For this review, take the finished solid that the model builds, in its own axes (mm). Face numbers are marked on the shaded views. A direction names the side the tool comes from. Round coordinates to 2 decimals unless told otherwise and drop trailing zeros. Order: outer loops, then holes, each group sorted by start corner. A loop starts at its lowest first (then second) coordinate and runs counter-clockwise, first axis right, second up. Notation, with made-up numbers: M 82,2.5 L 108,2.5 A16 cw 108,24.5 Z; hole C -23,79.25 d2. An arc over 180 degrees is marked long. Answer as a JSON object with one key per item and string values.
from build123d import *

# Parameters (mm, degrees)
BOSS_EXTRUDE3_DEPTH    = 370
SKETCH3_W              = 619.706220458
SKETCH3_H              = 524.5
BOSS_EXTRUDE4_DEPTH    = 50
BOSS_EXTRUDE6_DEPTH    = 420
CHAMFER1_SIZE          = 30
SHELL1_T               = -3.18
CUT_EXTRUDE1_DEPTH     = 10
BOSS_EXTRUDE7_REACH    = 652.082
SKETCH13_W             = 122.046220458
SKETCH13_H             = 233.985108613
CUT_EXTRUDE3_DEPTH     = 651.08233795
SPLIT2_SURFACE_1_BACK  = 938.174
SPLIT2_SURFACE_1_DEPTH = 1876.348
BOSS_EXTRUDE8_DEPTH    = 3.18


with BuildPart() as part:
    # Sketch1 → Boss-Extrude3 (new body)
    with BuildSketch(Plane(origin=(0, 0, 0), x_dir=(1, 0, 0), z_dir=(0, 1, 0))):
        Polygon((225.65, -262.25), (394.056220458, -262.25), (394.056220458, 262.25), (225.65, 262.25), (-225.65, 262.25), (-225.65, -262.25), align=None)
    extrude(amount=BOSS_EXTRUDE3_DEPTH)

    # Sketch3 → Boss-Extrude4 (add)
    with BuildSketch(Plane(origin=(0, 370, 0), x_dir=(1, 0, 0), z_dir=(0, 1, 0))):
        with Locations((84.203110229, 0)):
            Rectangle(SKETCH3_W, SKETCH3_H)
    extrude(amount=BOSS_EXTRUDE4_DEPTH)

    # Sketch9 → Boss-Extrude6 (add)
    with BuildSketch(Plane(origin=(0, 0, 0), x_dir=(1, 0, 0), z_dir=(0, 1, 0))):
        Polygon((-225.65, -262.25), (-152.747945688, -301.540612909), (321.154166146, -301.540612909), (394.056220458, -262.25), align=None)
    extrude(amount=BOSS_EXTRUDE6_DEPTH)

    # Chamfer1
    chamfer1_edges = [part.edges().sort_by_distance(p)[0] for p in [
        (-189.198972844, 420, 281.895306454),
        (84.203110229, 420, 301.540612909),
        (357.605193302, 420, 281.895306454),
    ]]
    chamfer(chamfer1_edges, length=CHAMFER1_SIZE)

    # Shell1
    shell1_openings = [part.faces().sort_by_distance(p)[0] for p in [
        (84.203110229, 0, 17.423394881),
    ]]
    offset(amount=SHELL1_T, openings=shell1_openings, kind=Kind.INTERSECTION)

    # Sketch7 → Cut-Extrude1 (cut)
    with BuildSketch(Plane.ZY.offset(225.65)):
        Polygon((-19.07, 315), (-19.07, 230), (20.93, 190), (80.93, 190), (120.93, 230), (120.93, 315), align=None)
    extrude(amount=-CUT_EXTRUDE1_DEPTH, mode=Mode.SUBTRACT)


with BuildPart() as body_2:

    # Sketch12 → Boss-Extrude7 (new, up to next)
    with BuildSketch(Plane(origin=(0, 0, 0), x_dir=(1, 0, 0), z_dir=(0, 1, 0)), mode=Mode.PRIVATE) as boss_extrude7_sk1:
        Polygon((225.65, -262.25), (225.65, -298.360612909), (320.351791074, -298.360612909), (390.876220458, -260.35142261), (390.876220458, 259.07), (225.65, 259.07), align=None)
    boss_extrude7_tool1 = extrude(boss_extrude7_sk1.sketch, amount=BOSS_EXTRUDE7_REACH, mode=Mode.PRIVATE) - part.part
    add(boss_extrude7_tool1.solids().sort_by_distance((307.390302, 0, 15.716589))[0])

    # Sketch13 → Cut-Extrude3 (cut, through all)
    with BuildSketch(Plane.XZ):
        with Locations((289.853110229, 233.456942929)):
            Rectangle(SKETCH13_W, SKETCH13_H)
    extrude(amount=-CUT_EXTRUDE3_DEPTH, mode=Mode.SUBTRACT)


with BuildPart() as part_1:
    add(part.part)

    # Split2: cut with a surface, the side it looks to stays
    # Split2 surface: a surface, the sketch's curves swept straight by 1876.348 mm
    with BuildLine(Plane.ZY.offset(225.65).offset(-SPLIT2_SURFACE_1_BACK), mode=Mode.PRIVATE) as split2_surface_1_path:
        Line((377.982656301, 50), (20.93, 50))
        Line((20.93, 50), (-30.817816509, 101.747816509))
        Line((-30.817816509, 101.747816509), (-303.707153017, 101.747816509))
    split2_surface_1 = Shell.extrude(split2_surface_1_path.wire(), (-1 * SPLIT2_SURFACE_1_DEPTH, 0 * SPLIT2_SURFACE_1_DEPTH, 0 * SPLIT2_SURFACE_1_DEPTH))
    split(bisect_by=split2_surface_1, keep=Keep.TOP)

    add(body_2.part)  # Boss-Extrude8 merges body 2
    # Sketch14 → Boss-Extrude8 (add)
    with BuildSketch(Plane.XZ):
        Polygon((394.056220458, 262.25), (394.056220458, -262.25), (-225.65, -262.25), (-225.65, 262.25), (-152.747945688, 301.540612909), (321.154166146, 301.540612909), align=None)
    extrude(amount=BOSS_EXTRUDE8_DEPTH)


solid = part_1.part
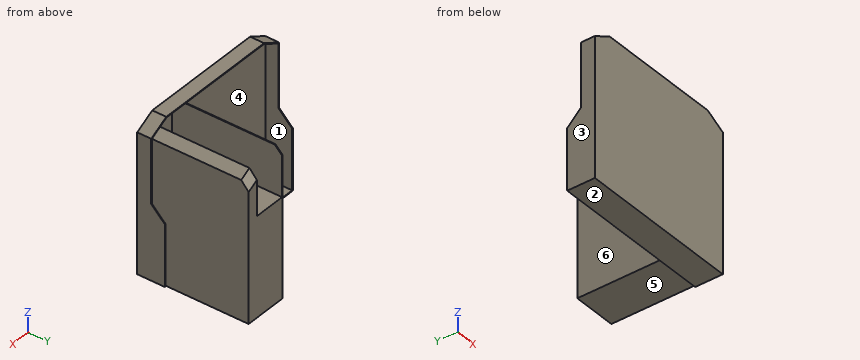
1) Add section B-B on z = 64. State the section outline as (x, y) points.
Geometry check:
{"outline": "M -225.65,-3.18 L 394.06,-3.18 L 394.06,50 L 390.88,50 L 390.88,416.82 L 225.65,416.82 L 225.65,0 L -222.47,0 L -222.47,50 L -225.65,50 Z"}
2) Machinability: for the marked faces 1 and 2, which of the approach directions +Z, -Z, +X, -X, +Y, -Y give a long, thin tool a straight path to every point of the face, cutting with its end or side? Answer none if there is none.
Geometry check:
{"face 1": "+Y", "face 2": "-Z, +X, -X, +Y, -Y"}
3) For L1, parallel to Z at x = 65, y = 19.5; L2, parallel to X at y = 36, z = -109.5; L3, parallel to Z at x = -33, y = 71, list the stretches that pass through material, from the lowest coordinate up.
Geometry check:
{"L1": "z = -262.25 to -259.07, 298.36 to 301.54", "L2": "x = -225.65 to -222.47, 225.65 to 394.06", "L3": "z = -262.25 to -259.07"}
4) Add section A-A on y = 40. State the section outline as (x, z) points.
Geometry check:
{"outline": "M -225.65,-262.25 L 394.06,-262.25 L 394.06,262.25 L 321.15,301.54 L -152.75,301.54 L -225.65,262.25 Z; hole M -222.47,-259.07 L 225.65,-259.07 L 225.65,298.36 L -151.95,298.36 L -222.47,260.35 Z; hole M 228.83,116.46 L 350.88,116.46 L 350.88,281.91 L 320.35,298.36 L 228.83,298.36 Z"}
5) Add section D-D on x = 243.5. State the section outline as (y, z) points, and give its area (3 significant figures).
Geometry check:
{"outline": "M -3.18,-262.25 L 101.75,-262.25 L 101.75,-259.07 L 416.82,-259.07 L 416.82,116.46 L 0,116.46 L 0,298.36 L 50,298.36 L 50,301.54 L -3.18,301.54 Z", "area": "159,000 mm²"}
6) Insertion check: P1, Ø1.5, axis at x = 315, y = 86, coming from the +Z side; P2, Ø4, axis at y = 228.5, z = -77.5, coming from the +X side; P3, Ø3, axis at y = 319.5, z = -173.5, coming from the -X side. Each pin has a flat end and moves straight along its axis. Give the tip position at first contact, or say it passes through.
Geometry check:
{"P1": "stops at z = 116.46", "P2": "stops at x = 390.88", "P3": "stops at x = 225.65"}
7) Mouldability with a two-part tool opening along X and no side actions: class the marked faces 3, 4, 5 and 6 as +X half, -X half, draft (parallel to the pull), parting line (faces both ways), or undercut.
Geometry check:
{"face 3": "-X half", "face 4": "undercut", "face 5": "draft", "face 6": "undercut"}
8) Add section C-C on y = 172.5. State the section outline as (x, z) points, and give its area (3 significant figures).
Geometry check:
{"outline": "M 225.65,-259.07 L 390.88,-259.07 L 390.88,260.35 L 350.88,281.91 L 350.88,116.46 L 228.83,116.46 L 228.83,298.36 L 225.65,298.36 Z", "area": "68,800 mm²"}
